```python
from build123d import *

# Parameters (mm, degrees)
SKETCH1_W                   = 17
SKETCH1_H                   = 17
BOSS_EXTRUDE1_DEPTH         = 1220
CUT_EXTRUDE1_START          = -20
SKETCH2_W                   = 20
SKETCH2_H                   = 20
CUT_EXTRUDE1_DEPTH          = 10
CUT_EXTRUDE2_DEPTH          = 15
SKETCH4_W                   = 3
SKETCH4_H                   = 10
CUT_EXTRUDE3_DEPTH          = 10
SKETCH_PATTERN1_START       = -20
SKETCH_PATTERN1_DEPTH       = 15
SKETCH_PATTERN1_2_OUTLINE_W = 1.5
SKETCH_PATTERN1_2_OUTLINE_H = 10
SKETCH_PATTERN1_2_DEPTH     = 3


# Read off the part's stored shape, not the designer's step: Sketch-Pattern1
with BuildPart() as part:
    # Sketch1 → Boss-Extrude1 (new body)
    with BuildSketch(Plane(origin=(0, 0, 0), x_dir=(1, 0, 0), z_dir=(0, 1, 0))):
        with BuildLine():
            Line((0.5, 0), (19.5, 0))
            ThreePointArc((19.5, 0), (19.853553391, 0.146446609), (20, 0.5))
            Line((20, 0.5), (20, 19.5))
            ThreePointArc((20, 19.5), (19.853553391, 19.853553391), (19.5, 20))
            Line((19.5, 20), (0.5, 20))
            ThreePointArc((0.5, 20), (0.146446609, 19.853553391), (0, 19.5))
            Line((0, 19.5), (0, 0.5))
            ThreePointArc((0, 0.5), (0.146446609, 0.146446609), (0.5, 0))
        make_face()
        with Locations((10, 10)):
            Rectangle(SKETCH1_W, SKETCH1_H, mode=Mode.SUBTRACT)
    extrude(amount=BOSS_EXTRUDE1_DEPTH)

    # Sketch2 → Cut-Extrude1 (cut)
    with BuildSketch(Plane(origin=(20, 0, 0), x_dir=(0, 0, -1), z_dir=(1, 0, 0)).offset(CUT_EXTRUDE1_START)):
        with Locations((10, 1210)):
            Rectangle(SKETCH2_W, SKETCH2_H)
        with Locations((10, 10)):
            Rectangle(SKETCH2_W, SKETCH2_H)
    extrude(amount=CUT_EXTRUDE1_DEPTH, mode=Mode.SUBTRACT)

    # Sketch3 → Cut-Extrude2 (cut)
    with BuildSketch(Plane(origin=(0, 0, -20), x_dir=(-1, 0, 0), z_dir=(0, 0, -1))):
        Polygon((-15, 1115), (0, 1115), (0, 1120), (-9, 1120), (-9, 1130), (0, 1130), (0, 1135), (-15, 1135), align=None)
    extrude(amount=-CUT_EXTRUDE2_DEPTH, mode=Mode.SUBTRACT)

    # Sketch4 → Cut-Extrude3 (cut)
    with BuildSketch(Plane.ZY):
        with Locations((-18.5, 1125)):
            Rectangle(SKETCH4_W, SKETCH4_H)
    extrude(amount=-CUT_EXTRUDE3_DEPTH, mode=Mode.SUBTRACT)

    # Sketch-Pattern1 outline → Sketch-Pattern1 (cut)
    with BuildSketch(Plane.XY.offset(SKETCH_PATTERN1_START)):
        Polygon((15, 85), (15, 105), (0, 105), (0, 100), (1.5, 100), (1.5, 90), (0, 90), (0, 85), align=None)
        Polygon((1.5, 330), (1.5, 320), (0, 320), (0, 315), (15, 315), (15, 335), (0, 335), (0, 330), align=None)
        Polygon((1.5, 500), (1.5, 490), (0, 490), (0, 485), (15, 485), (15, 505), (0, 505), (0, 500), align=None)
        Polygon((1.5, 730), (1.5, 720), (0, 720), (0, 715), (15, 715), (15, 735), (0, 735), (0, 730), align=None)
        Polygon((1.5, 900), (1.5, 890), (0, 890), (0, 885), (15, 885), (15, 905), (0, 905), (0, 900), align=None)
    extrude(amount=SKETCH_PATTERN1_DEPTH, mode=Mode.SUBTRACT)

    # Sketch-Pattern1 2 outline → Sketch-Pattern1 2 (cut)
    with BuildSketch(Plane.XY.offset(SKETCH_PATTERN1_START)):
        with Locations((0.75, 95)):
            Rectangle(SKETCH_PATTERN1_2_OUTLINE_W, SKETCH_PATTERN1_2_OUTLINE_H)
        with Locations((0.75, 325)):
            Rectangle(SKETCH_PATTERN1_2_OUTLINE_W, SKETCH_PATTERN1_2_OUTLINE_H)
        with Locations((0.75, 495)):
            Rectangle(SKETCH_PATTERN1_2_OUTLINE_W, SKETCH_PATTERN1_2_OUTLINE_H)
        with Locations((0.75, 725)):
            Rectangle(SKETCH_PATTERN1_2_OUTLINE_W, SKETCH_PATTERN1_2_OUTLINE_H)
        with Locations((0.75, 895)):
            Rectangle(SKETCH_PATTERN1_2_OUTLINE_W, SKETCH_PATTERN1_2_OUTLINE_H)
    extrude(amount=SKETCH_PATTERN1_2_DEPTH, mode=Mode.SUBTRACT)


solid = part.part
```
Can you work these out from the model? Positions are in its coordinate system, mm. Coordinates: 2 decimals unless noted, no trailing zeros. Loops run counter-clockwise (first coordinate to the right, second up) from the corner with the lowest first, then second, coordinate; pieces in that order, holes last. Notation, with made-up numbers: (-25.5, 4) -> (-15.5, 4) arc R16 ccw to (-15.5, 17) -> close; hole circle Ø8 at (32.5, 65.5). An arc over 180 degrees is marked (long way). Answer as a JSON object with one key per item and string values.
1) For P1, Ø0.8, axis at x = 1, y = 503, coming from the -Z side; P2, Ø12, axis at x = 5.5, z = -12, coming from the +Y side; P3, Ø1.2, axis at x = 1, y = 1124.5, coming from the -Z side; P4, Ø10, axis at x = 16, z = -14, coming from the -Y side, each with a flat end and sliding along its axis, tell me the tip position at first contact or that it passes through.
Results:
{"P1": "stops at z = -5", "P2": "stops at y = 1200", "P3": "stops at z = -17", "P4": "stops at y = 0"}
2) If I drill on line 1 (Z direction, x = 4.75, y = 274.5); line 2 (X direction, y = 1101, z = -11), over which ranges is the centre line in solid material (lowest first)?
Results:
{"line 1": "z = -20 to -18.5, -1.5 to 0", "line 2": "x = 0 to 1.5, 18.5 to 20"}
3) Imagine slicing it at B-B (y = 813.5). Please give me the cut outline in (x, z), then the cut area to 3 significant figures.
Results:
{"outline": "(0, -19.5) arc R0.5 ccw to (0.5, -20) -> (19.5, -20) arc R0.5 ccw to (20, -19.5) -> (20, -0.5) arc R0.5 ccw to (19.5, 0) -> (0.5, 0) arc R0.5 ccw to (0, -0.5) -> close; hole (1.5, -18.5) -> (18.5, -18.5) -> (18.5, -1.5) -> (1.5, -1.5) -> close", "area": "111 mm^2"}
4) Imagine slicing it at A-A (x = 6.25). Count the separate pieces of the cut face and the enclosed holes in it, then the cut area to 3 significant figures.
Results:
{"separate pieces": "8", "enclosed holes": "0", "area": "3,360 mm^2"}
